Solid Edge part; units mm, degrees
sketch "Sketch1" plane through (0, 0, 0) normal (0, -1, 0) x (1, 0, 0)
  line L0 (1.5, 0) -> (3, 1.5)
  line L1 (3, 1.5) -> (3, 1.7)
  line L2 (3, 1.7) -> (0, 1.7)
  line L3 (0, 1.7) -> (0, -10.3)
  line L4 (0, -10.3) -> (1.1935, -10.3)
  line L5 (1.1935, -10.3) -> (1.5, -9.9935)
  line L6 (1.5, -9.9935) -> (1.5, -1.5)
  line L7 (1.5, -1.5) -> (1.1935, -1.5)
  line L8 (1.1935, -1.5) -> (1.1935, -1.49)
  line L9 (1.1935, -1.49) -> (1.5, -1.49)
  line L10 (1.5, -1.49) -> (1.5, 0)
  dimension "D1" = 1.5
  dimension "D2" = 1.1935
revolve "RevolvedProtrusion1" add sketch "Sketch1" angle 360 about axis through (0, 0, 54) along (0, 0, -1)
sketch "Sketch2" plane through (0, 0, 0) normal (0, -1, 0) x (1, 0, 0)
  arc A0 (-1, 0.5) -> (0, 0) centre (0, 1.25) ccw
  line L0 (0, 0.5) -> (0, 0)
  line L1 (-1, 0.5) -> (0, 0.5)
revolve "RevolvedCutout1" cut sketch "Sketch2" angle 360 about axis through (0, 0, 54) along (0, 0, -1)
sketch "Sketch3" plane through (0, 0, 1.7) normal (0, 0, 1) x (0, -1, 0)
  line L0 (-1.1547, 0) -> (-0.5774, 1)
  line L1 (-0.5774, 1) -> (0.5774, 1)
  line L2 (0.5774, 1) -> (1.1547, 0)
  line L3 (1.1547, 0) -> (0.5774, -1)
  line L4 (0.5774, -1) -> (-0.5774, -1)
  line L5 (-0.5774, -1) -> (-1.1547, 0)
extrude "Cutout1" cut sketch "Sketch3" against normal blind 1.2
cosmetic_thread "Thread1"
sketch "Sketch4" plane through (0, 0, 0) normal (1, 0, 0) x (0, 1, 0)
  line L0 (-1.15, 1.7) -> (0, 1.036)
revolve "RevolvedCutout2" cut sketch "Sketch4" angle 360 about axis through (0, 0, -57) along (0, 0, 1) material side at (0, -0.55, 1.4113)
fillet "Round1" radius 0.1 1 edges at (-1.5, 0, 0)
properties material "Steel"
Source: CAD feature listing. Evaluate the final solid. Frame: model axes, mm. A direction names the side the tool comes from. Coordinates: 2 decimals unless noted, no trailing zeros. Write each loop counter-clockwise with the first axis right and the second up, starting at its lowest first coordinate (ties: lowest second). Pieces come first, ordered by that corner, then holes. Notation, with made-up numbers: (-32.75, 21.5) -> (-6.75, 21.5) arc R16 cw to (-6.75, 48.5) -> close; hole circle Ø6 at (13.5, -1). An arc over 180 degrees is marked (long way). Return JSON: item names as keys, results as strings. Group by question number.
1) Set-up query: faces 4 (the face through (-1.5, 0.07, -0.76)), 5 (the face through (0.51, -0.86, 1.11)), 6 (the face through (0, 0, -10.3)). Return all of +Z, -Z, +X, -X, +Y, -Y with unobstructed straight access to the full face (end or side cutting, diameter ignored); none if empty.
2) Mould query, pull axis Y, two halves, no side actions, for faces 1 (the face through (-1.5, 0.07, -5.69)), 2 (the face through (-0.51, 0.86, 1.11)), 3 (the face through (1.3, 0, 1.7)). Classes: +Y half, -Y half, draft (parallel to the pull), parting line (faces both ways), or undercut.
3) Section query A-A, the plane z = -5.5. Return loops of the section in (x, y).
4) Contact query for flat-ended pins moving along their axis: P1, Ø1, axis at x = -1.5, y = -1.5, coming from the -Z side; P2, Ø0.9, axis at x = 0, y = -0.5, coming from the +Z side; P3, Ø1.5, axis at x = -1.5, z = -6.5, coming from the -Y side. Output: stop coordinate, or through.
5) Ray query, line 1 along Y through (x, z) = (0, -8.75); line 2 along Z through (x, y) = (2.5, -1); line 3 along Z through (x, y) = (0, 2.5). Return the intervals inside material, ascending.
From the geometry:
{
 "1": {"face 4": "-Z", "face 5": "+Z", "face 6": "-Z, +X, -X, +Y, -Y"},
 "2": {"face 1": "parting line", "face 2": "undercut", "face 3": "draft"},
 "3": {"outline": "circle Ø3 at (0, 0)"},
 "4": {"P1": "z = 0.12", "P2": "z = 0.44", "P3": "y = -1.3"},
 "5": {"line 1": "-1.5 to 1.5", "line 2": "1.19 to 1.7", "line 3": "1 to 1.7"}
}
